from build123d import *

# Parameters (mm, degrees)
F1_DEPTH = 2.8
F3_DEPTH = 0.2
F5_DEPTH = 0.2


with BuildPart() as f1:
    # F0 (on Top) → F1 (new body)
    with BuildSketch(Plane.XY):
        with BuildLine():
            ThreePointArc((-41.5, -23.65), (-39.640128, -28.140128), (-35.15, -30))
            Line((-35.15, -30), (35.15, -30))
            ThreePointArc((35.15, -30), (39.640128, -28.140128), (41.5, -23.65))
            Line((41.5, -23.65), (41.5, -0.635))
            ThreePointArc((41.5, -0.635), (43.359872, 3.855128), (47.85, 5.715))
            Line((47.85, 5.715), (59.405295, 5.715))
            ThreePointArc((59.405295, 5.715), (64.511092, 8.28964), (65.476545, 13.925759))
            Line((65.476545, 13.925759), (61.925894, 25.510759))
            ThreePointArc((61.925894, 25.510759), (59.630003, 28.755797), (55.854644, 30))
            Line((55.854644, 30), (41.5, 30))
            Line((41.5, 30), (-35.15, 30))
            ThreePointArc((-35.15, 30), (-39.640128, 28.140128), (-41.5, 23.65))
            Line((-41.5, 23.65), (-41.5, -23.65))
        make_face()
    extrude(amount=F1_DEPTH)

    # F2 (on face) → F3 (cut)
    with BuildSketch(Plane.XY.offset(2.8)):
        with BuildLine():
            ThreePointArc((39.5, -0.635), (41.945658, 5.269342), (47.85, 7.715))
            Line((47.85, 7.715), (59.405295, 7.715))
            ThreePointArc((59.405295, 7.715), (62.902967, 9.47873), (63.56434, 13.339693))
            Line((63.56434, 13.339693), (60.013689, 24.924693))
            ThreePointArc((60.013689, 24.924693), (58.440914, 27.147672), (55.854644, 28))
            Line((55.854644, 28), (-35.15, 28))
            ThreePointArc((-35.15, 28), (-38.225914, 26.725914), (-39.5, 23.65))
            Line((-39.5, 23.65), (-39.5, -23.65))
            ThreePointArc((-39.5, -23.65), (-38.225914, -26.725914), (-35.15, -28))
            Line((-35.15, -28), (35.15, -28))
            ThreePointArc((35.15, -28), (38.225914, -26.725914), (39.5, -23.65))
            Line((39.5, -23.65), (39.5, -0.635))
        make_face()
    extrude(amount=-F3_DEPTH, mode=Mode.SUBTRACT)

    # F4 (on face) → F5 (cut)
    with BuildSketch(Plane(origin=(0, 0, 0), x_dir=(1, 0, 0), z_dir=(0, 0, -1))):
        with BuildLine():
            ThreePointArc((-39.5, -23.65), (-38.225914, -26.725914), (-35.15, -28))
            Line((-35.15, -28), (55.854644, -28))
            ThreePointArc((55.854644, -28), (58.440914, -27.147672), (60.013689, -24.924693))
            Line((60.013689, -24.924693), (63.56434, -13.339693))
            ThreePointArc((63.56434, -13.339693), (62.902967, -9.47873), (59.405295, -7.715))
            Line((59.405295, -7.715), (47.85, -7.715))
            ThreePointArc((47.85, -7.715), (41.945658, -5.269342), (39.5, 0.635))
            Line((39.5, 0.635), (39.5, 23.65))
            ThreePointArc((39.5, 23.65), (38.225914, 26.725914), (35.15, 28))
            Line((35.15, 28), (-35.15, 28))
            ThreePointArc((-35.15, 28), (-38.225914, 26.725914), (-39.5, 23.65))
            Line((-39.5, 23.65), (-39.5, -23.65))
        make_face()
    extrude(amount=-F5_DEPTH, mode=Mode.SUBTRACT)


solid = f1.part
The listing builds one solid part. Answer for the finished solid, in the listing's coordinates (mm). A direction names the side the tool comes from. Give positions to 0.01 mm unless a question says otherwise; leave off trailing zeros. Order: outer loops, then holes, each group sorted by start corner. A loop starts at its lowest first (then second) coordinate and runs counter-clockwise, first axis right, second up. Notation, with made-up numbers: (4.5, -10.5) -> (47.5, -10.5) arc R29 ccw to (47.5, 24.5) -> close; hole circle Ø5 at (-1, 36.5). An arc over 180 degrees is marked (long way). Put each result on its own line as item: value.
Item 1: Given P1, Ø1.4, axis at y = -9, z = 2, coming from the +X side; P2, Ø2, axis at x = 30, y = 10.5, coming from the +Z side; P3, Ø1.4, axis at x = 54.5, z = 1.5, coming from the -Y side (3 decimals), each flat-ended and moving along its own axis, determine where each tip first touches the part or whether it passes through.
Established:
P1: stops at x = 41.5
P2: stops at z = 2.6
P3: stops at y = 5.715
Item 2: A cutting plane is placed at B-B on x = 52.5. Give the vertices of the cut face in (y, z) (3 decimals).
Established:
outline: (5.715, 0) -> (7.715, 0) -> (7.715, 0.2) -> (28, 0.2) -> (28, 0) -> (30, 0) -> (30, 2.8) -> (28, 2.8) -> (28, 2.6) -> (7.715, 2.6) -> (7.715, 2.8) -> (5.715, 2.8) -> close
Item 3: A cutting plane is placed at A-A on z = 1.5. Give the vertices of the cut face in (x, y) (3 decimals).
Established:
outline: (-41.5, -23.65) arc R6.35 ccw to (-35.15, -30) -> (35.15, -30) arc R6.35 ccw to (41.5, -23.65) -> (41.5, -0.635) arc R6.35 cw to (47.85, 5.715) -> (59.405, 5.715) arc R6.35 ccw to (65.477, 13.926) -> (61.926, 25.511) arc R6.35 ccw to (55.855, 30) -> (-35.15, 30) arc R6.35 ccw to (-41.5, 23.65) -> close
Item 4: For a pull along X with two mould halves and no side action, classify faces 1 (the face through (-39.69, -28.09, 1.38)), 2 (the face through (0, 0, 2.6)), 3 (the face through (59.68, 28.72, 1.38)), 4 (the face through (0, -30, 1)) as released by +X, released by -X, zero draft, split by the parting line, or undercut.
Established:
face 1: released by -X
face 2: undercut
face 3: released by +X
face 4: zero draft
Item 5: For faces 5 (the face through (54, 5.715, 1)), 6 (the face through (-39.59, 28.19, 1.38)), determine the directions among +Z, -Z, +X, -X, +Y, -Y from which every point of the face is accessible in a straight line to the end or side of a thin tool.
Established:
face 5: +Z, -Z, +X, -Y
face 6: +Z, -Z, -X, +Y
Item 6: Straight lines are drawn through the part: line 1 (X direction, y = -17, z = 1.3); line 2 (Z direction, x = -5, y = 23); line 3 (Y direction, x = 52, z = 1.55) (3 decimals). For each, find the intervals that lie inside material, in ascending order.
Established:
line 1: x = -41.5 to 41.5
line 2: z = 0.2 to 2.6
line 3: y = 5.715 to 30
